from build123d import *

# Parameters (mm, degrees)
F0_R     = 40
F0_R_2   = 5.0000025111
F0_R_3   = 2.5
F1_DEPTH = 2
F2_R     = 5
F2_R_2   = 2.5
F3_DEPTH = 5
F4_R     = 2.49999
F5_R     = 0.99999


# Not quite as in the source:
# - a fillet or chamfer is up to 0.001 mm smaller than in the source, because OpenCascade refuses the exact size


with BuildPart() as f1:
    # F0 (on Front) → F1 (new body)
    with BuildSketch(Plane.XZ):
        Circle(F0_R)
        with Locations((-8.4519767052, -28.7847892084)):
            Circle(F0_R_2, mode=Mode.SUBTRACT)
        with Locations((-22.6724872306, -19.6458220184)):
            Circle(F0_R_2, mode=Mode.SUBTRACT)
        with Locations((-29.6946432564, -4.2694451482)):
            Circle(F0_R_2, mode=Mode.SUBTRACT)
        with Locations((8.4519767052, -28.7847892084)):
            Circle(F0_R_2, mode=Mode.SUBTRACT)
        with Locations((22.6724872306, -19.6458220184)):
            Circle(F0_R_2, mode=Mode.SUBTRACT)
        with Locations((29.6946432564, -4.2694451482)):
            Circle(F0_R_2, mode=Mode.SUBTRACT)
        with Locations((-27.2889598606, 12.4624503901)):
            Circle(F0_R_2, mode=Mode.SUBTRACT)
        with Locations((-16.2192245237, 25.2376059849)):
            Circle(F0_R_2, mode=Mode.SUBTRACT)
        Circle(F0_R_3, mode=Mode.SUBTRACT)
        with Locations((27.2889598606, 12.4624503901)):
            Circle(F0_R_2, mode=Mode.SUBTRACT)
        with Locations((16.2192245237, 25.2376059849)):
            Circle(F0_R_2, mode=Mode.SUBTRACT)
        with Locations((0, 30)):
            Circle(F0_R_2, mode=Mode.SUBTRACT)
    extrude(amount=F1_DEPTH)

    # F2 (on Front) → F3 (join)
    with BuildSketch(Plane.XZ):
        Circle(F2_R)
        Circle(F2_R_2, mode=Mode.SUBTRACT)
    extrude(amount=-F3_DEPTH)

    # F4 (radius 2.5 in the source; OpenCascade refuses exactly that, so slightly less here)
    f4_edges = [f1.edges().sort_by_distance(p)[0] for p in [
        (-5, 0, 0),
        (-5, 5, 0),
    ]]
    fillet(f4_edges, radius=F4_R)

    # F5 (radius 1 in the source; OpenCascade refuses exactly that, so slightly less here)
    f5_edges = [f1.edges().sort_by_distance(p)[0] for p in [
        (40, -1, 0),
        (-40, 0, 0),
        (-40, -2, 0),
    ]]
    fillet(f5_edges, radius=F5_R)


solid = f1.part
Check sheet for the modelled part. Datum: model origin and axes. Units: mm. Coordinates: 2 decimals unless noted, no trailing zeros. Answer in a Markdown table with one row per item.
1. Material ranges on line 1 along X through (y, z) = (-0.5, -31.5); line 2 along Y through (x, z) = (-33.5, -9.5); line 3 along X through (y, z) = (-0.5, 1.5), recorded low to high. Write a range as [from, to].
Check values:
| item | result |
|---|---|
| line 1 | x = [-24.43, -12.65], [-4.25, 4.25], [12.65, 24.43] |
| line 2 | y = [-2, 0] |
| line 3 | x = [-39.84, -2], [2, 39.84] |
2. Release check for a two-part mould opening along X. For faces 1 (the face through (8, -2, 1)), 2 (the face through (29.977, -0.986, 16.678)) record: released by +X, released by -X, zero draft, split by the parting line, or undercut.
Check values:
| item | result |
|---|---|
| face 1 | zero draft |
| face 2 | undercut |
3. Sectioned sample at A-A, the plane x = 0. Give the number of separate pieces and of enclosed holes in the cut face, then the cut area to 3 significant figures.
Check values:
| item | result |
|---|---|
| separate pieces | 3 |
| enclosed holes | 0 |
| area | 154 mm2 |
4. Go/stop test with flat-tipped pins: pin 1 (6.5 mm diameter, centred on x = 0, z = 0, fed in from -Y); pin 2 (11.5 mm diameter, centred on x = 27.29, z = 12.46, fed in from +Y); pin 3 (12 mm diameter, centred on x = 10.5, z = -5, fed in from +Y). Record where each tip stops, or that it passes through.
Check values:
| item | result |
|---|---|
| pin 1 | stops at y = -2 |
| pin 2 | stops at y = 0 |
| pin 3 | stops at y = 0.84 |
